Input: dimensioned drawing with shaded views. Units: mm. Origin: part minimum x, y, z. Coordinates: 2 decimals unless noted, no trailing zeros. Order: outer loops, then holes, each group sorted by start corner. A loop starts at its lowest first (then second) coordinate and runs counter-clockwise, first axis right, second up. Notation, with made-up numbers: (42, 12) - (68, 12) arc R4 ccw to (68, 16) - close; hole circle Ø3 at (-20.75, 34.5). An arc over 180 degrees is marked (long way). Use one line per item in the form item = value. Start each with the question number.
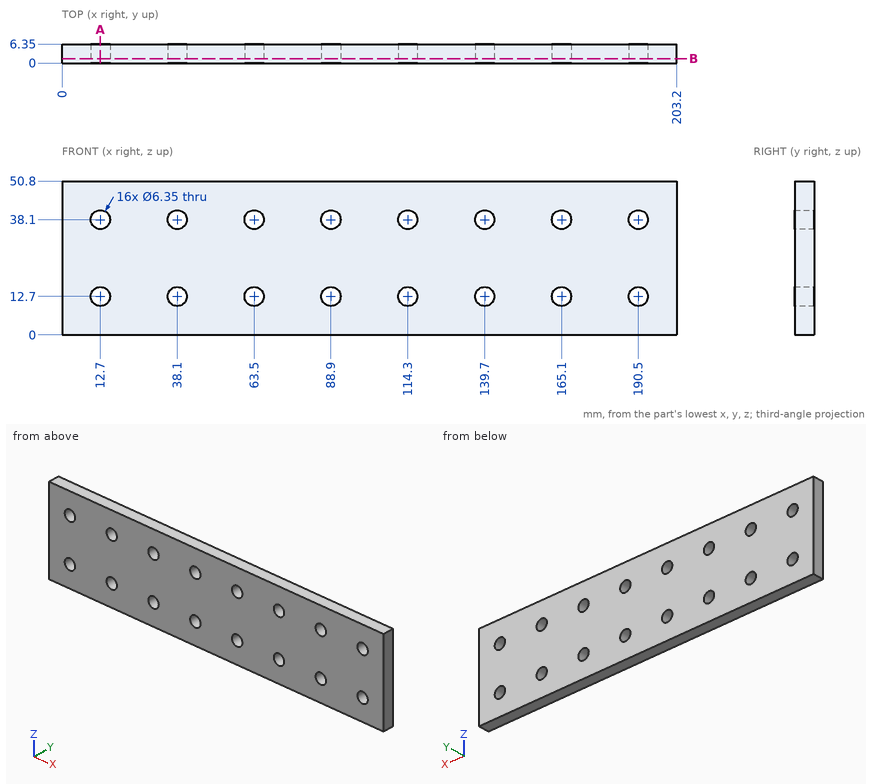
(1) Contact query for a flat-ended pin moving along its axis: pin 1 Ø7.5 at (x, z) = (114.3, 38.1) entering from +Y. Output: stop coordinate, or through.
(2) Material intervals for L1, parallel to Z at x = 190.5, y = 3.25 (3 decimals); L2, parallel to Z at x = 138, y = 1, sorted ascending. Write a range as from..to.
(3) Cut plane B-B on y = 1.5. Count the separate pieces of the cut face and the enclosed holes in it, plus the area to 3 significant figures.
(4) Cut plane A-A on x = 12.7. Return the cut outline in (y, z) (3 decimals).
Check sheet entries:
q1.pin_1 = 6.35
q2.L1 = 0..9.525, 15.875..34.925, 41.275..50.8
q2.L2 = 0..10.02, 15.38..35.42, 40.78..50.8
q3.separate_pieces = 1
q3.enclosed_holes = 16
q3.area = 9,820 mm^2
q4.outline = (0, 0) - (6.35, 0) - (6.35, 9.525) - (0, 9.525) - close; (0, 15.875) - (6.35, 15.875) - (6.35, 34.925) - (0, 34.925) - close; (0, 41.275) - (6.35, 41.275) - (6.35, 50.8) - (0, 50.8) - close
